Verification items for the finished model (mm, model axes). Face numbers are marked on the shaded views. A direction names the side the tool comes from. Give positions to 0.01 mm unless a question says otherwise; leave off trailing zeros. Order: outer loops, then holes, each group sorted by start corner. A loop starts at its lowest first (then second) coordinate and runs counter-clockwise, first axis right, second up.
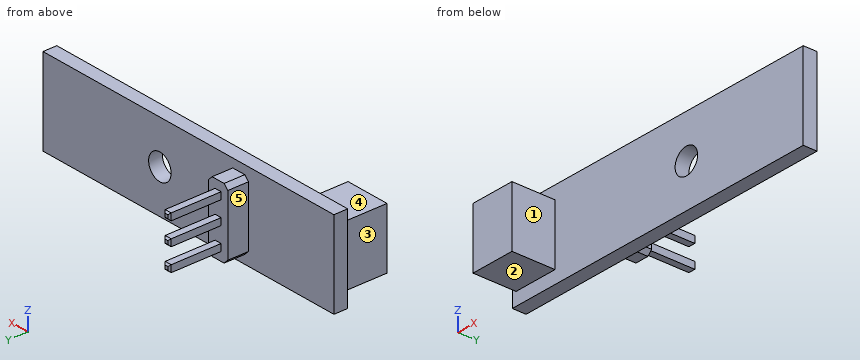
Autodesk Inventor part; units mm, degrees
ref_plane "YZ Plane" through (0, 0, 0) normal (1, 0, 0) x (0, 1, 0)
ref_plane "XZ Plane" through (0, 0, 0) normal (0, 1, 0) x (-1, 0, 0)
ref_plane "XY Plane" through (0, 0, 0) normal (0, 0, 1) x (1, 0, 0)
sketch "Эскиз2" plane through (0, 0, 0) normal (0, 1, 0) x (-1, 0, 0)
  line L0 (0, 0) -> (38.3359, 0) construction
  line L1 (38.3359, 0) -> (38.3359, -10) construction
  line L2 (38.3359, -10) -> (0, -10) construction
  line L3 (0, -10) -> (0, 0) construction
  line L4 (0, 0) -> (38.3359, 0)
  line L5 (38.3359, 0) -> (38.3359, -10)
  line L6 (38.3359, -10) -> (0, -10)
  line L7 (0, -10) -> (0, 0)
  circle A0 centre (15.6, -5) radius 1.5
  point P0 (0, -5)
  dimension "d1" = 10
  dimension "d11" = 15.6
  dimension "d12" = 3
extrude "Выдавливание1" add sketch "Эскиз2" along normal blind 1.6
sketch "Эскиз3" plane through (0, 1.6, 0) normal (0, 1, 0) x (1, 0, 0)
  line L0 (0, 0) -> (-38.3359, 0) construction
  line L1 (-38.3359, 0) -> (-38.3359, 10) construction
  line L2 (-38.3359, 10) -> (0, 10) construction
  line L3 (0, 10) -> (0, 0) construction
  line L4 (-27.4359, 9) -> (-24.8359, 9)
  line L5 (-24.8359, 9) -> (-24.8359, 1)
  line L6 (-24.8359, 1) -> (-27.4359, 1)
  line L7 (-27.4359, 1) -> (-27.4359, 9)
  point P0 (-27.4359, 5)
  point P1 (-38.3359, 5)
  dimension "d43" = 2.6
  dimension "d50" = 8
  dimension "d51" = 10.9
extrude "Выдавливание2" add sketch "Эскиз3" along normal blind 2.4
chamfer "Фаска1" distance 0.5 angle 45 4 edges at (-24.8359, 2.8, -1) (-27.4359, 2.8, -1) (-24.8359, 2.8, -9) (-27.4359, 2.8, -9)
sketch "Эскиз4" plane through (0, 4, 0) normal (0, 1, 0) x (1, 0, 0)
  line L0 (-26.5359, 8) -> (-25.7359, 8)
  line L1 (-25.7359, 8) -> (-25.7359, 7.2)
  line L2 (-25.7359, 7.2) -> (-26.5359, 7.2)
  line L3 (-26.5359, 7.2) -> (-26.5359, 8)
  line L4 (-26.5359, 5.4) -> (-25.7359, 5.4)
  line L5 (-25.7359, 5.4) -> (-25.7359, 4.6)
  line L6 (-25.7359, 4.6) -> (-26.5359, 4.6)
  line L7 (-26.5359, 4.6) -> (-26.5359, 5.4)
  line L8 (-26.5359, 2) -> (-25.7359, 2)
  line L9 (-25.7359, 2) -> (-25.7359, 2.8)
  line L10 (-25.7359, 2.8) -> (-26.5359, 2.8)
  line L11 (-26.5359, 2.8) -> (-26.5359, 2)
  line L12 (-27.4359, 8.5) -> (-26.9359, 9)
  line L13 (-27.4359, 8.5) -> (-27.4359, 1.5)
  line L14 (-26.9359, 1) -> (-27.4359, 1.5)
  line L15 (-26.9359, 1) -> (-25.3359, 1)
  line L16 (-24.8359, 1.5) -> (-25.3359, 1)
  line L17 (-24.8359, 1.5) -> (-24.8359, 8.5)
  line L18 (-25.3359, 9) -> (-24.8359, 8.5)
  line L19 (-25.3359, 9) -> (-26.9359, 9)
  line L20 (-27.4359, 5) -> (-24.8359, 5)
  point P0 (0, 0)
  point P1 (-26.5359, 5)
  point P2 (-26.1359, 5.4)
  point P3 (-26.1359, 9)
  dimension "d57" = 0.8
  dimension "d58" = 4.4
extrude "Выдавливание3" add sketch "Эскиз4" along normal blind 6 contours L0 L1 L2 L3 | L4 L5 L20 L7 | L20 L5 L6 L7 | L11 L10 L9 L8
chamfer "Фаска2" distance 0.2 angle 45 12 edges at (-26.1359, 10, -2) (-26.5359, 10, -2.4) (-26.1359, 10, -2.8) (-25.7359, 10, -2.4) (-26.1359, 10, -4.6) (-26.5359, 10, -5) (-26.1359, 10, -5.4) (-25.7359, 10, -5) (-26.1359, 10, -7.2) (-26.5359, 10, -7.6) (-26.1359, 10, -8) (-25.7359, 10, -7.6)
sketch "Эскиз5" plane through (0, 0, 0) normal (0, -1, 0) x (1, 0, 0)
  line L0 (-38.3359, -8.5) -> (-33.1359, -8.5)
  line L1 (-33.1359, -8.5) -> (-33.1359, -1.5)
  line L2 (-33.1359, -1.5) -> (-38.3359, -1.5)
  line L3 (-38.3359, -1.5) -> (-38.3359, -8.5)
  line L4 (-38.3359, 0) -> (-38.3359, -10)
  line L5 (0, -10) -> (-38.3359, -10) construction
  line L6 (-38.3359, -10) -> (-38.3359, 0) construction
  line L7 (-38.3359, 0) -> (0, 0) construction
  line L8 (0, 0) -> (0, -10) construction
  point P0 (0, 0)
  point P1 (-38.3359, -5)
  point P2 (-38.3359, -5)
  dimension "d106" = 5.2
  dimension "d109" = 7
sketch "Эскиз6" plane through (-38.3359, 0, -10) normal (-1, 0, 0) x (0, 0, 1)
  line L0 (10, 0) -> (0, 0)
  line L1 (10, 0) -> (10, 1.6)
  line L2 (0, 1.6) -> (10, 1.6)
  line L3 (0, 0) -> (0, 1.6)
  point P0 (10, 0)
extrude "Выдавливание4" add sketch "Эскиз6" along normal blind 0.5
extrude "Выдавливание5" add sketch "Эскиз5" along normal blind 5
properties part number "LineSensor"
(1) Section check A-A, the plane x = -15.6. Enter the section's corners in (y, z).
Solved:
outline: (0, -10) - (1.6, -10) - (1.6, -6.5) - (0, -6.5) - close; (0, -3.5) - (1.6, -3.5) - (1.6, 0) - (0, 0) - close
(2) Section check B-B, the plane y = 5.5. Enter the section's corners in (x, z), then the cut area to 3 significant figures.
Solved:
outline: (-26.54, -8) - (-25.74, -8) - (-25.74, -7.2) - (-26.54, -7.2) - close; (-26.54, -5.4) - (-25.74, -5.4) - (-25.74, -4.6) - (-26.54, -4.6) - close; (-26.54, -2.8) - (-25.74, -2.8) - (-25.74, -2) - (-26.54, -2) - close
area: 1.92 mm2
(3) Set-up check for the marked faces 1, 2, 3, 4 and 5: record each of +Z, -Z, +X, -X, +Y, -Y from which the full face is reachable in a straight line by a thin tool's end or side.
Solved:
face 1: +Z, -Z, +X, -Y
face 2: -Z, +X, -X, -Y
face 3: +Z, -Z, -X, -Y
face 4: +Z, +X, -X, -Y
face 5: +Z, -Z, -X, +Y
(4) Section check D-D, the plane y = -0.75. Enter the section's corners in (x, z).
Solved:
outline: (-38.34, -8.5) - (-33.14, -8.5) - (-33.14, -1.5) - (-38.34, -1.5) - close
(5) Scan lines: line 1 (Z direction, x = -26, y = 8); line 2 (Z direction, x = -15.6, y = 0.6); line 3 (Y direction, x = -33.5, z = -4.75). Record each from-to range of solid material in increasing order.
Solved:
line 1: z = -8 to -7.2, -5.4 to -4.6, -2.8 to -2
line 2: z = -10 to -6.5, -3.5 to 0
line 3: y = -5 to 1.6
(6) Go/stop test with flat-tipped pins: pin 1 (3 mm diameter, centred on x = -14.5, z = -2.5, fed in from -Y); pin 2 (0.9 mm diameter, centred on y = 7, z = -5, fed in from -X); pin 3 (0.9 mm diameter, centred on x = -26, y = 6.5, fed in from +Z). Record where each tip stops, or that it passes through.
Solved:
pin 1: stops at y = 0
pin 2: stops at x = -26.54
pin 3: stops at z = -2
(7) Section check C-C, the plane x = -9.5. Enter the section's corners in (y, z).
Solved:
outline: (0, -10) - (1.6, -10) - (1.6, 0) - (0, 0) - close
